For this review, use the dimensioned drawing (mm, ordinates from the lowest corner) and the shaded views. A direction names the side the tool comes from. Coordinates: 2 decimals unless noted, no trailing zeros. Loops run counter-clockwise (first coordinate to the right, second up) from the corner with the lowest first, then second, coordinate; pieces in that order, holes last. Notation, with made-up numbers: (0, 24) -> (51, 24) arc R10 cw to (51, 34) -> close; hole circle Ø5 at (23, -12). An arc over 180 degrees is marked (long way). Answer as a JSON object with one key per item and string values.
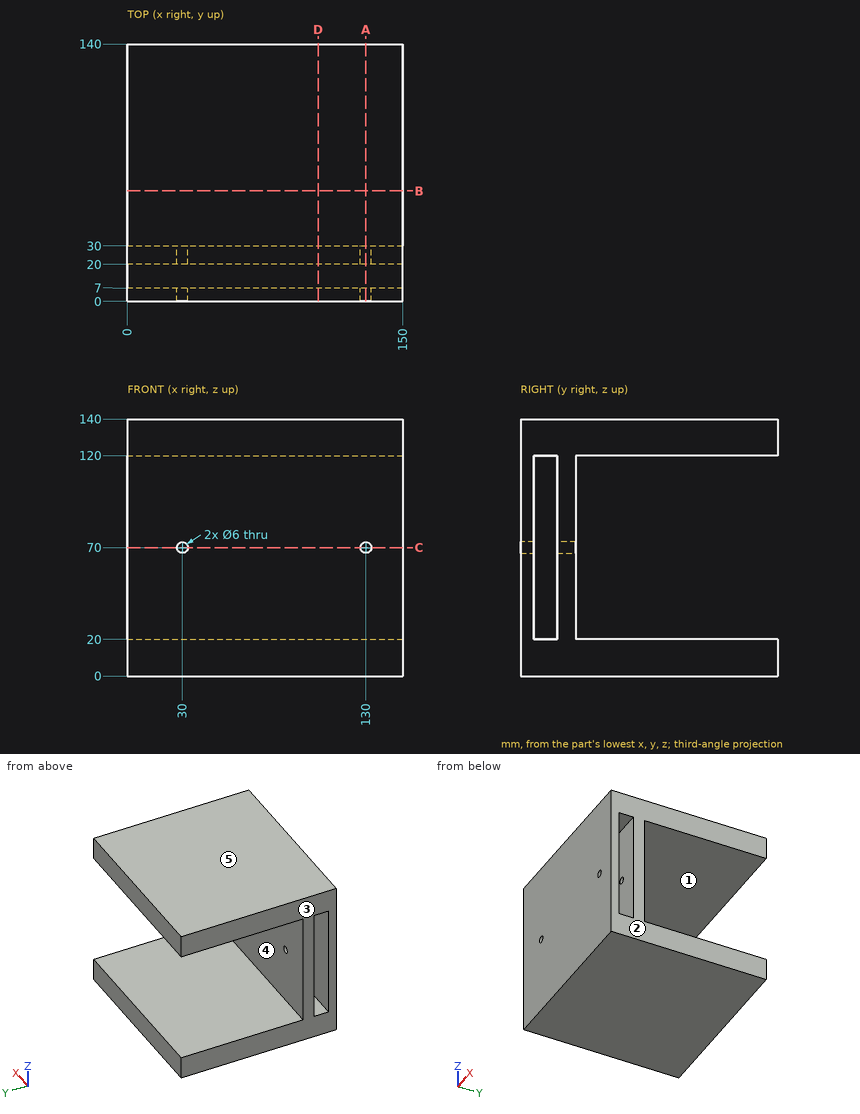
1) The part is to be moulded in two halves that separate along Z. For the marked faces 3, 4 and 5, say which applies: pulls with the +Z half, pulls with the -Z half, needs draft (parallel to the pull), parting line crosses it, or undercut.
Completed:
{"face 3": "needs draft", "face 4": "undercut", "face 5": "pulls with the +Z half"}
2) Add section A-A, the plane x = 130. Give the boundary of the cut face in (y, z).
Completed:
{"outline": "(0, 0) -> (140, 0) -> (140, 20) -> (30, 20) -> (30, 67) -> (20, 67) -> (20, 20) -> (7, 20) -> (7, 67) -> (0, 67) -> close; (0, 73) -> (7, 73) -> (7, 120) -> (20, 120) -> (20, 73) -> (30, 73) -> (30, 120) -> (140, 120) -> (140, 140) -> (0, 140) -> close"}
3) Add section D-D, the plane x = 104. Give the boundary of the cut face in (y, z), and give its area (3 significant figures).
Completed:
{"outline": "(0, 0) -> (140, 0) -> (140, 20) -> (30, 20) -> (30, 120) -> (140, 120) -> (140, 140) -> (0, 140) -> close; hole (7, 20) -> (20, 20) -> (20, 120) -> (7, 120) -> close", "area": "7,300 mm²"}
4) Clearance check with flat-ended pins moving along their axes: pin 1 Ø8 at (x, z) = (30, 70) entering from +Y; pin 2 Ø6 at (x, z) = (29, 61) entering from -Y. State where each tip first meets the part, or that it passes through.
Completed:
{"pin 1": "y = 30", "pin 2": "y = 0"}
5) Wall thickness on probe 1 along X at (y, z) = (3, 70); probe 2 along Y at (x, z) = (96, 89.5); probe 3 along Z at (x, y) = (10, 58): over which ranges is each line inside the solid? List them lowest first.
Completed:
{"probe 1": "0 to 27, 33 to 127, 133 to 150", "probe 2": "0 to 7, 20 to 30", "probe 3": "0 to 20, 120 to 140"}
6) Add section B-B, the plane y = 60. Give the boundary of the cut face in (x, z), and give its area (3 significant figures).
Completed:
{"outline": "(0, 0) -> (150, 0) -> (150, 20) -> (0, 20) -> close; (0, 120) -> (150, 120) -> (150, 140) -> (0, 140) -> close", "area": "6,000 mm²"}
7) Add section C-C, the plane z = 70. Give the boundary of the cut face in (x, y), and give its area (3 significant figures).
Completed:
{"outline": "(0, 0) -> (27, 0) -> (27, 7) -> (0, 7) -> close; (0, 20) -> (27, 20) -> (27, 30) -> (0, 30) -> close; (33, 0) -> (127, 0) -> (127, 7) -> (33, 7) -> close; (33, 20) -> (127, 20) -> (127, 30) -> (33, 30) -> close; (133, 0) -> (150, 0) -> (150, 7) -> (133, 7) -> close; (133, 20) -> (150, 20) -> (150, 30) -> (133, 30) -> close", "area": "2,350 mm²"}
8) For the marked faces 1 and 2, list the 3-axis set-ups (+Z, -Z, +X, -X, +Y, -Y) from which the entire face can be reached by the end or side of a thin tool; tool diameter is ignored.
Completed:
{"face 1": "+X, -X, +Y", "face 2": "+Z, -Z, +X, +Y, -Y"}
